```python
from build123d import *

# Parameters (mm, degrees)
SKETCH1_R           = 3
BOSS_EXTRUDE1_DEPTH = 3


with BuildPart() as part:
    # Sketch1 → Boss-Extrude1 (new body)
    with BuildSketch(Plane(origin=(0, 0, 0), x_dir=(0, 1, 0), z_dir=(0, 0, 1))):
        with BuildLine():
            Line((-0.823178029, 4.367911471), (22.959093686, -56.487309327))
            ThreePointArc((22.959093686, -56.487309327), (23.036789975, -58.446570398), (21.887628759, -60.035333804))
            ThreePointArc((21.887628759, -60.035333804), (-9.269367484, -69.787393269), (-40.327126668, -59.723762055))
            ThreePointArc((-40.327126668, -59.723762055), (-41.576105768, -57.134789232), (-40.074300788, -54.683807619))
            ThreePointArc((-40.074300788, -54.683807619), (-22.12312602, -32.858554253), (-23.076923077, -4.615384615))
            ThreePointArc((-23.076923077, -4.615384615), (-16.491925767, 11.12756051), (-0.823178029, 4.367911471))
        make_face()
        with Locations(Location((-12, 6, 0), (0, 0, 270))):
            Circle(SKETCH1_R, mode=Mode.SUBTRACT)
        with Locations(Location((-12, -6, 0), (0, 0, 270))):
            Circle(SKETCH1_R, mode=Mode.SUBTRACT)
    extrude(amount=BOSS_EXTRUDE1_DEPTH)


solid = part.part
```
Geometry check sheet. Reference: the model listing, model coordinates, mm. Round coordinates to 2 decimals unless told otherwise and drop trailing zeros. Order: outer loops, then holes, each group sorted by start corner. A loop starts at its lowest first (then second) coordinate and runs counter-clockwise, first axis right, second up. Notation, with made-up numbers: (16.25, 78.5) - (42.25, 78.5) arc R13 cw to (42.25, 101.5) - close; hole circle Ø2 at (76.5, 76.25). An arc over 180 degrees is marked (long way). Use a Markdown table: item, result. Add a question column.
1) Thickness scan on line 1 along Y through (x, z) = (-6, 1.55); line 2 along Y through (x, z) = (6, 2.1); line 3 along X through (y, z) = (-32.5, 2.5). Record the ranges inside material, lowest first.
2) Section check C-C (y = -12). Record the cut outline in (x, z).
3) Mould release check, pull along X, two halves, no side actions. Record for faces 1 (the cylindrical face through (8.77, -13.15, 1.48)), 2 (the cylindrical face through (58.42, 23.045, 1.479)), 3 (the cylindrical face through (69.788, -8.805, 1.479)): released by +X, released by -X, zero draft, split by the parting line, or undercut.
4) Gauge pin test, flat end, axial feed: P1, Ø1, axis at x = 44, z = 2, coming from the -Y side. Record the tip position at first contact, or that the pin passes through.
5) Section check D-D (x = -6). Record the cut outline in (y, z).
6) Section check B-B (z = 2.05). Record the cut outline in (x, y), then the cut area to 3 significant figures.
7) Section check A-A (x = 6). Record the cut outline in (y, z), then the cut area to 3 significant figures.
Established:
| question | item | result |
|---|---|---|
| 1 | line 1 | -22.39 to -15, -9 to -1.61 |
| 1 | line 2 | -22.53 to -15, -9 to 3.23 |
| 1 | line 3 | 49.05 to 64.38 |
| 2 | outline | (-12, 0) - (-9, 0) - (-9, 3) - (-12, 3) - close; (-3, 0) - (3, 0) - (3, 3) - (-3, 3) - close; (9, 0) - (69.7, 0) - (69.7, 3) - (9, 3) - close |
| 3 | face 1 | undercut |
| 3 | face 2 | split by the parting line |
| 3 | face 3 | released by +X |
| 4 | P1 | y = -28.38 |
| 5 | outline | (-22.39, 0) - (-15, 0) - (-15, 3) - (-22.39, 3) - close; (-9, 0) - (-1.61, 0) - (-1.61, 3) - (-9, 3) - close |
| 6 | outline | (-4.37, -0.82) arc R12 ccw (long way) to (4.62, -23.08) arc R40 cw to (54.68, -40.07) arc R3 ccw to (59.72, -40.33) arc R53.79 ccw to (60.04, 21.89) arc R3 ccw to (56.49, 22.96) - close; hole circle Ø6 at (-6, -12); hole circle Ø6 at (6, -12) |
| 6 | area | 2,880 mm2 |
| 7 | outline | (-22.53, 0) - (-15, 0) - (-15, 3) - (-22.53, 3) - close; (-9, 0) - (3.23, 0) - (3.23, 3) - (-9, 3) - close |
| 7 | area | 59.3 mm2 |
